The listing builds one solid part. Answer for the finished solid, in the listing's coordinates (mm). A direction names the side the tool comes from. Round coordinates to 2 decimals unless told otherwise and drop trailing zeros. Write each loop counter-clockwise with the first axis right and the second up, starting at its lowest first coordinate (ties: lowest second). Pieces come first, ordered by that corner, then holes.
from build123d import *

# Parameters (mm, degrees)
PAD008_DEPTH               = 0.5
PAD009_DEPTH               = 0.5
PAD009_MIRRORED004_2_DEPTH = 0.5
SKETCH021_W                = 1.5
SKETCH021_H                = 1
PAD010_DEPTH               = 0.75
SKETCH021_MIRRORED006_2_W  = 1.5
SKETCH021_MIRRORED006_2_H  = 1
PAD010_MIRRORED006_2_DEPTH = 0.75
FILLET_R                   = 0.25
FILLET001_R                = 0.25
FILLET003_R                = 0.49


with BuildPart() as part:
    # Sketch018 → Pad008 (new body)
    with BuildSketch(Plane.XY.offset(13)):
        Polygon((-1, 6), (-1, 6.7), (-4.5, 6.7), (-5.118749, 5), (-5.5, 5), (-5.5, -5), (-5.118749, -5), (-4.5, -6.7), (4.5, -6.7), (5.118749, -5), (5.5, -5), (5.5, 5), (5.118749, 5), (4.5, 6.7), (1, 6.7), (1, 6), align=None)
    extrude(amount=-PAD008_DEPTH)

    # Sketch020 → Pad009 (join)
    with BuildSketch(Plane.YZ.offset(6)):
        Polygon((-5, 13), (-5, 2.368609), (-4.131391, 1.5), (-1, 1.5), (0, 1.5), (0, 13), align=None)
    pad009 = extrude(amount=-PAD009_DEPTH)

    # Sketch020 Mirrored004 2 → Pad009 Mirrored004 2 (add)
    with BuildSketch(Plane.YZ.offset(-6)):
        Polygon((-5, 13), (-5, 2.368609), (-4.131391, 1.5), (-1, 1.5), (0, 1.5), (0, 13), align=None)
    pad009_mirrored004_2 = extrude(amount=PAD009_MIRRORED004_2_DEPTH)

    # Mirrored005: Pad009, Pad009 Mirrored004 2 across XZ
    add(pad009.mirror(Plane.XZ))
    add(pad009_mirrored004_2.mirror(Plane.XZ))

    # Sketch021 → Pad010 (join)
    with BuildSketch(Plane.XY.offset(1.5)):
        with Locations((-5.25, 1.5)):
            Rectangle(SKETCH021_W, SKETCH021_H)
    pad010 = extrude(amount=-PAD010_DEPTH)

    # Sketch021 Mirrored006 2 → Pad010 Mirrored006 2 (add)
    with BuildSketch(Plane(origin=(0, 0, 1.5), x_dir=(-1, 0, 0), z_dir=(0, 0, -1))):
        with Locations((-5.25, 1.5)):
            Rectangle(SKETCH021_MIRRORED006_2_W, SKETCH021_MIRRORED006_2_H)
    pad010_mirrored006_2 = extrude(amount=PAD010_MIRRORED006_2_DEPTH)

    # Mirrored007: Pad010, Pad010 Mirrored006 2 across XZ
    add(pad010.mirror(Plane.XZ))
    add(pad010_mirrored006_2.mirror(Plane.XZ))

    # Fillet
    fillet_edges = [part.edges().sort_by_distance(p)[0] for p in [
        (-6, -1.5, 0.75),
        (-6, 1.5, 0.75),
        (6, 1.5, 0.75),
        (6, -1.5, 0.75),
    ]]
    fillet(fillet_edges, radius=FILLET_R)

    # Fillet001
    fillet001_edges = [part.edges().sort_by_distance(p)[0] for p in [
        (6, 0, 13),
        (-6, 0, 13),
    ]]
    fillet(fillet001_edges, radius=FILLET001_R)

    # Fillet003
    fillet003_edges = [part.edges().sort_by_distance(p)[0] for p in [
        (4.5, 2, 1.125),
        (4.5, 1, 1.125),
        (4.5, -1, 1.125),
        (4.5, -2, 1.125),
        (-4.5, -2, 1.125),
        (-4.5, -1, 1.125),
        (-4.5, 1, 1.125),
        (-4.5, 2, 1.125),
    ]]
    fillet(fillet003_edges, radius=FILLET003_R)


solid = part.part
1. Straight lines are drawn through the part: line 1 along X through (y, z) = (0, 5.5); line 2 along Z through (x, y) = (-1.25, -2.25). For each, find the intervals that lie inside material, in ascending order.
Geometry says:
line 1: x = -6 to -5.5, 5.5 to 6
line 2: z = 12.5 to 13
2. Section B-B on y = -4.5 is taken. Determine the outline of the cut face in (x, z), plus the area to 3 significant figures.
Geometry says:
outline: (-6, 1.87) - (-5.5, 1.87) - (-5.5, 12.5) - (5.5, 12.5) - (5.5, 1.87) - (6, 1.87) - (6, 12.75) arc R0.25 ccw to (5.75, 13) - (-5.75, 13) arc R0.25 ccw to (-6, 12.75) - close
area: 16.6 mm2
3. Given pin 1 (0.6 mm diameter, centred on y = 6.5, z = 13, fed in from +X); pin 2 (0.8 mm diameter, centred on x = -5.5, z = 1, fed in from -Y); pin 3 (5 mm diameter, centred on x = -4.5, y = 5, fed in from -Z), each flat-ended and moving along its own axis, determine where each tip first touches the part or whether it passes through.
Geometry says:
pin 1: stops at x = 4.68
pin 2: stops at y = -2
pin 3: stops at z = 1.5
4. Section A-A on z = 10 is taken. Determine the outline of the cut face in (x, y).
Geometry says:
outline: (-6, -5) - (-5.5, -5) - (-5.5, 5) - (-6, 5) - close; (5.5, -5) - (6, -5) - (6, 5) - (5.5, 5) - close
5. For a pull along Z with two mould halves and no side action, classify faces 3 (the face through (-5.75, -4.57, 1.94)), 4 (the face through (-5.8, -5, 7.8)), 5 (the face through (-5, -1.5, 1.5)) as released by +Z, released by -Z, zero draft, split by the parting line, or undercut.
Geometry says:
face 3: released by -Z
face 4: zero draft
face 5: undercut
6. Section D-D on y = -1.25 is taken. Determine the outline of the cut face in (x, z).
Geometry says:
outline: (-6, 1) arc R0.25 ccw to (-5.75, 0.75) - (-4.56, 0.75) - (-4.56, 1.5) - (-5.5, 1.5) - (-5.5, 12.5) - (5.5, 12.5) - (5.5, 1.5) - (4.56, 1.5) - (4.56, 0.75) - (5.75, 0.75) arc R0.25 ccw to (6, 1) - (6, 12.75) arc R0.25 ccw to (5.75, 13) - (-5.75, 13) arc R0.25 ccw to (-6, 12.75) - close
7. A tool of negligible diameter and unlimited length cuts with its end or side. For faces 1 (the face through (0, 0, 13)), 2 (the face through (5.5, 0, 7)), from which of +Z, -Z, +X, -X, +Y, -Y can it reach the whole face along a straight path? Write none if from no direction.
Geometry says:
face 1: +Z, +X, -X, +Y, -Y
face 2: +Y, -Y
8. Section C-C on x = 4 is taken. Determine the outline of the cut face in (y, z).
Geometry says:
outline: (-6.7, 12.5) - (6.7, 12.5) - (6.7, 13) - (-6.7, 13) - close
